Design review of the part built by this model. Coordinates are the model's own, in mm. A direction names the side the tool comes from. Give positions to 0.01 mm unless a question says otherwise; leave off trailing zeros. Loops run counter-clockwise (first coordinate to the right, second up) from the corner with the lowest first, then second, coordinate; pieces in that order, holes last. Notation, with made-up numbers: M 58,-9.75 L 106,-9.75 A35 ccw 106,26.25 Z; hole C 17.5,-30.75 d6. An arc over 180 degrees is marked long. Answer as CSV lines item,"result".
```python
from build123d import *

# Parameters (mm, degrees)
ESBO_O2_R             = 4
CORTE_EXTRUS_O1_DEPTH = 60
PADR_OCIRCULAR1_COUNT = 6


with BuildPart() as part:
    # Esboço1 → Revolução1 (revolve)
    with BuildSketch(Plane.XY):
        Polygon((35, 28.575), (38, 28.575), (38, 22.575), (29, 22.575), (29, 0), (24, 0), (24, 22.575), (0, 22.575), (0, 28.575), (32, 28.575), (32, 25.575), (35, 25.575), align=None)
    revolve(axis=Axis((0, 0, 0), (-1, 0, 0)))

    # Esboço2 → Corte-extrusão1 (cut)
    with BuildSketch(Plane.XY):
        with Locations((16, 0)):
            Circle(ESBO_O2_R)
    corte_extrus_o1 = extrude(amount=-CORTE_EXTRUS_O1_DEPTH, mode=Mode.SUBTRACT)

    # PadrãoCircular1: Corte-extrusão1 ×6 about axis
    padr_ocircular1_axis = Axis((0, 0, 0), (1, 0, 0))
    for i in range(1, PADR_OCIRCULAR1_COUNT):
        add(corte_extrus_o1.rotate(padr_ocircular1_axis, i * 360 / PADR_OCIRCULAR1_COUNT), mode=Mode.SUBTRACT)


solid = part.part
```
1. For faces 4 (the flat face through (29, 0, 0)), 5 (the cylindrical face through (11.83, -4.89, 22.04)), 6 (the cylindrical face through (33.521, -5.544, 24.967)), list the 3-axis set-ups (+Z, -Z, +X, -X, +Y, -Y) from which the entire face can be reached by the end or side of a thin tool; tool diameter is ignored.
Answer block:
face 4,"+X"
face 5,"-X"
face 6,"none"
2. The part is to be moulded in two halves that separate along Z. For faces 1 (the flat face through (35, 21, 15)), 2 (the cylindrical face through (33.44, -4.89, 22.04)), 3 (the cylindrical face through (36.521, -28.547, -1.256)), say which applies: pulls with the +Z half, pulls with the -Z half, needs draft (parallel to the pull), parting line crosses it, or undercut.
Answer block:
face 1,"needs draft"
face 2,"undercut"
face 3,"parting line crosses it"
3. We need section D-D, the plane x = 5. Write out the cut boundary in (y, z) (3 decimals).
Answer block:
outline,"C 0,0 d57.15; hole C 0,0 d45.15"
4. For P1, Ø5, axis at x = 20, z = -16, coming from the -Y side; P2, Ø1, axis at y = -20.5, z = -3, coming from the +X side; P3, Ø10, axis at x = 20.5, y = -11.5, coming from the +Z side, all flat-tipped, find the tip position at first contact; note any pin that passes through.
Answer block:
P1,"y = -25.18"
P2,"x = 29"
P3,"z = 27.83"
5. We need section B-B, the plane x = 14.5. Count the separate pieces of the cut face and the enclosed holes in it, plus the area to 3 significant figures.
Answer block:
separate pieces,"6"
enclosed holes,"0"
area,"696 mm²"
6. We need section A-A, the plane y = 0. Write out the cut boundary in (x, z) (3 decimals).
Answer block:
outline,"M 0,-28.575 L 12,-28.575 L 12,-22.575 L 0,-22.575 Z; M 0,22.575 L 12,22.575 L 12,28.575 L 0,28.575 Z; M 20,-28.575 L 32,-28.575 L 32,-25.575 L 35,-25.575 L 35,-28.575 L 38,-28.575 L 38,-22.575 L 29,-22.575 L 29,22.575 L 38,22.575 L 38,28.575 L 35,28.575 L 35,25.575 L 32,25.575 L 32,28.575 L 20,28.575 L 20,22.575 L 24,22.575 L 24,-22.575 L 20,-22.575 Z"
7. We need section C-C, the plane z = 0. Write out the cut boundary in (x, y) (3 decimals), plus the area to 3 significant figures.
Answer block:
outline,"M 0,-28.575 L 32,-28.575 L 32,-25.575 L 35,-25.575 L 35,-28.575 L 38,-28.575 L 38,-22.575 L 29,-22.575 L 29,22.575 L 38,22.575 L 38,28.575 L 35,28.575 L 35,25.575 L 32,25.575 L 32,28.575 L 0,28.575 L 0,22.575 L 24,22.575 L 24,-22.575 L 0,-22.575 Z"
area,"664 mm²"
8. To check wall thickness, follow L1, parallel to X at y = 0, z = -26.5; L2, parallel to Z at x = 8, y = 0.5; L3, parallel to Y at x = 8, z = 0 (3 decimals). State the ranges of each line that lie inside material, in increasing order. Write a range as [from, to].
Answer block:
L1,"[0, 12], [20, 32], [35, 38]"
L2,"[-28.57, -22.57], [22.57, 28.57]"
L3,"[-28.575, -22.575], [22.575, 28.575]"
